Check sheet for the drawn part. Datum: minimum x, y, z corner. Units: mm. A direction names the side the tool comes from. Give positions to 0.01 mm unless a question says otherwise; leave off trailing zeros. Loops run counter-clockwise (first coordinate to the right, second up) from the corner with the lowest first, then second, coordinate; pieces in that order, holes last.
1. Cross-section at D-D, the plane x = 40. Record the cut outline in (y, z).
2. Release check for a two-part mould opening along X. For the marked faces 6, 7 and 8 record: +X half, -X half, draft (parallel to the pull), parting line (faces both ways), or undercut.
3. Go/stop test with flat-tipped pins: pin 1 Ø1.3 at (y, z) = (5, 34) entering from +X; pin 2 Ø8.5 at (x, y) = (32, 5.5) entering from +Z; pin 3 Ø4.5 at (y, z) = (7, 30) entering from -X; pin 4 Ø4 at (x, y) = (56, 10) entering from +Z. Record where each tip stops, or that it passes through.
4. Cross-section at A-A, the plane z = 30. Record the cut outline in (x, y) (3 decimals).
5. Tool access check on the marked faces 1, 2, 3, 4 and 5. Record the directions out of +Z, -Z, +X, -X, +Y, -Y that give a thin tool (end or side, any length) a straight path to the whole face; none if there is none.
6. Cross-section at B-B, the plane y = 7.25. Record the cut outline in (x, z) (3 decimals).
7. Material ranges on L1, parallel to X at y = 2.25, z = 24.5 (3 decimals); L2, parallel to Z at x = 62.5, y = 13.5; L3, parallel to Z at x = 43, y = 6.75, recorded low to high.
8. Cross-section at C-C, the plane x = 24. Record the cut outline in (y, z).
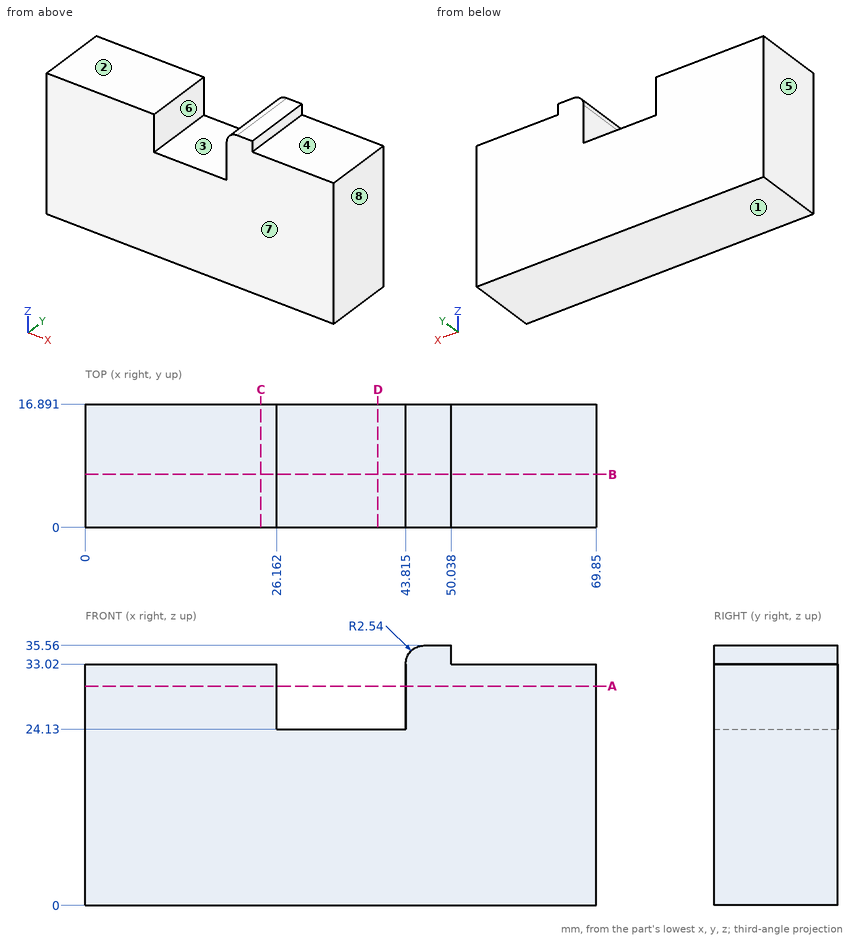
Result:
1. outline: (0, 0) - (16.89, 0) - (16.89, 24.13) - (0, 24.13) - close
2. face 6: undercut
2. face 7: draft
2. face 8: +X half
3. pin 1: stops at x = 50.04
3. pin 2: stops at z = 24.13
3. pin 3: stops at x = 0
3. pin 4: stops at z = 33.02
4. outline: (0, 0) - (26.162, 0) - (26.162, 16.891) - (0, 16.891) - close; (43.815, 0) - (69.85, 0) - (69.85, 16.891) - (43.815, 16.891) - close
5. face 1: -Z, +X, -X, +Y, -Y
5. face 2: +Z, -X, +Y, -Y
5. face 3: +Z, +Y, -Y
5. face 4: +Z, +X, +Y, -Y
5. face 5: +Z, -Z, -X, +Y, -Y
6. outline: (0, 0) - (69.85, 0) - (69.85, 33.02) - (50.038, 33.02) - (50.038, 35.56) - (46.355, 35.56) arc R2.54 ccw to (43.815, 33.02) - (43.815, 24.13) - (26.162, 24.13) - (26.162, 33.02) - (0, 33.02) - close
7. L1: x = 0 to 26.162, 43.815 to 69.85
7. L2: z = 0 to 33.02
7. L3: z = 0 to 24.13
8. outline: (0, 0) - (16.89, 0) - (16.89, 33.02) - (0, 33.02) - close
